```python
from build123d import *

# Parameters (mm, degrees)
SKETCH1_W           = 370
SKETCH1_H           = 70
BOSS_EXTRUDE1_DEPTH = 10
SKETCH2_W           = 10
SKETCH2_H           = 20
BOSS_EXTRUDE2_DEPTH = 10
CUT_EXTRUDE1_DEPTH  = 199.368344249


with BuildPart() as part:
    # Sketch1 → Boss-Extrude1 (new body)
    with BuildSketch(Plane(origin=(0, 0, 0), x_dir=(1, 0, 0), z_dir=(0, 1, 0))):
        Rectangle(SKETCH1_W, SKETCH1_H)
    extrude(amount=BOSS_EXTRUDE1_DEPTH)

    # Sketch2 → Boss-Extrude2 (add, through all)
    with BuildSketch(Plane(origin=(0, 10, 0), x_dir=(1, 0, 0), z_dir=(0, 1, 0))):
        with Locations((190, 25)):
            Rectangle(SKETCH2_W, SKETCH2_H)
        with Locations((190, -25)):
            Rectangle(SKETCH2_W, SKETCH2_H)
    boss_extrude2 = extrude(amount=-BOSS_EXTRUDE2_DEPTH)

    # Sketch3 → Cut-Extrude1 (cut, through all)
    with BuildSketch(Plane(origin=(0, 10, 0), x_dir=(1, 0, 0), z_dir=(0, 1, 0))):
        with BuildLine():
            Line((185, -1.55), (185, 1.55))
            Line((185, 1.55), (180.5, 1.55))
            Line((180.5, 1.55), (180.5, 2.35))
            ThreePointArc((180.5, 2.35), (180.353553391, 2.703553391), (180, 2.85))
            Line((180, 2.85), (177.5, 2.85))
            ThreePointArc((177.5, 2.85), (177.146446609, 2.703553391), (177, 2.35))
            Line((177, 2.35), (177, 1.55))
            Line((177, 1.55), (174, 1.55))
            Line((174, 1.55), (174, -1.55))
            Line((174, -1.55), (177, -1.55))
            Line((177, -1.55), (177, -2.35))
            ThreePointArc((177, -2.35), (177.146446609, -2.703553391), (177.5, -2.85))
            Line((177.5, -2.85), (180, -2.85))
            ThreePointArc((180, -2.85), (180.353553391, -2.703553391), (180.5, -2.35))
            Line((180.5, -2.35), (180.5, -1.55))
            Line((180.5, -1.55), (185, -1.55))
        make_face()
    cut_extrude1 = extrude(amount=-CUT_EXTRUDE1_DEPTH, mode=Mode.SUBTRACT)

    # Mirror1: Boss-Extrude2, Cut-Extrude1 across plane
    add(boss_extrude2.mirror(Plane(origin=(0, 0, 0), x_dir=(0, 0, 1), z_dir=(1, 0, 0))))
    add(cut_extrude1.mirror(Plane(origin=(0, 0, 0), x_dir=(0, 0, 1), z_dir=(1, 0, 0))), mode=Mode.SUBTRACT)


solid = part.part
```
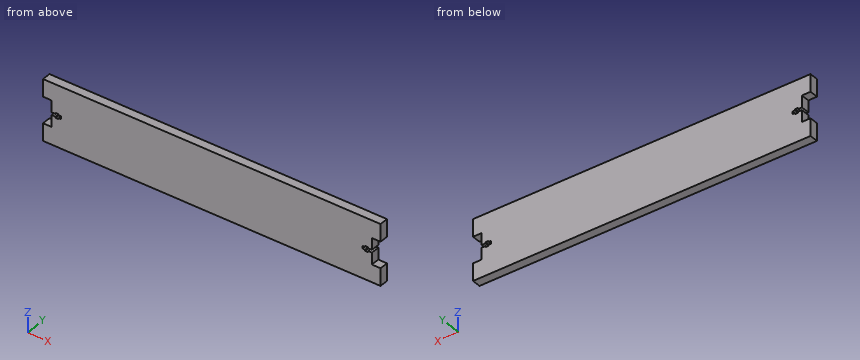
Read the model definition and answer for the solid it produces. Units are mm, in the model's axes. Coordinates: 2 decimals unless noted, no trailing zeros. Write each loop counter-clockwise with the first axis right and the second up, starting at its lowest first coordinate (ties: lowest second). Pieces come first, ordered by that corner, then holes. Notation, with made-up numbers: (-27.5, -26) -> (8.5, -26) arc R23 cw to (8.5, 2) -> close; hole circle Ø2 at (4, -31.75). An arc over 180 degrees is marked (long way). Answer as a JSON object with one key per item and string values.
Q1. Flat-ended cylindrical pins translate along their axes: pin 1 Ø0.9 at (y, z) = (3.5, 0.5) entering from +X; pin 2 Ø0.9 at (y, z) = (5.5, 2) entering from +X; pin 3 Ø0.9 at (y, z) = (4.5, -2) entering from -X. Find the tip coordinate at first contact, or state that the pin passes through.
The answers:
{"pin 1": "stops at x = 174", "pin 2": "stops at x = 185", "pin 3": "stops at x = -185"}
Q2. Consider line 1 (X direction, y = 4.5, z = 9); line 2 (X direction, y = 3.75, z = 1). Determine where each line is inside the solid, lowest interval first. Write a range as [from, to].
The answers:
{"line 1": "x = [-185, 185]", "line 2": "x = [-174, 174]"}
Q3. The part is cut by section A-A on z = 9.5. Give the vertices of the cut face in (x, y), then the cut area to 3 significant figures.
The answers:
{"outline": "(-185, 0) -> (185, 0) -> (185, 10) -> (-185, 10) -> close", "area": "3,700 mm2"}
